```python
from build123d import *

# Parameters (mm, degrees)
CROQUIS4_OUTSIDE_W    = 60.478
CROQUIS4_OUTSIDE_H    = 60.478
CORTAR_EXTRUIR6_DEPTH = 70
CROQUIS5_OUTSIDE_W    = 188.422
CROQUIS5_OUTSIDE_H    = 183.78
CROQUIS5_OUTSIDE_R    = 15
CORTAR_EXTRUIR7_DEPTH = 70
CORTAR_EXTRUIR7_TAPER = 45
CROQUIS6_R            = 9
CORTAR_EXTRUIR8_DEPTH = 15
CHAFL_N1_SIZE         = 2
REDONDEO1_R           = 1
CROQUIS7_OUTSIDE_W    = 83.062
CROQUIS7_OUTSIDE_H    = 78.42
CROQUIS7_OUTSIDE_R    = 15
CORTAR_EXTRUIR9_DEPTH = 10
CORTAR_EXTRUIR9_TAPER = 60


with BuildPart() as part:
    # Croquis1 → Revolución1 (revolve)
    with BuildSketch(Plane.XY):
        Polygon((6.35, 31.379194031), (20, 31.379194031), (22, 31.379194031), (22, 29.379194031), (22, 14.379194031), (22, 12.379194031), (20, 12.379194031), (14, 12.379194031), (11.11, 12.379194031), (11.11, 9.379194031), (9.525, -5.620805969), (1.5875, -5.620805969), (1.5875, 12.379194031), (6.35, 12.379194031), align=None)
    revolve(axis=Axis((0, 51.930492424, 0), (0, -1, 0)))

    # Croquis4 outside → Cortar-Extruir6 (cut)
    with BuildSketch(Plane(origin=(0, 31.379194031, 0), x_dir=(1, 0, 0), z_dir=(0, 1, 0))):
        Rectangle(CROQUIS4_OUTSIDE_W, CROQUIS4_OUTSIDE_H)
        Polygon((17.320508076, 0), (8.660254038, 15), (-8.660254038, 15), (-17.320508076, 0), (-8.660254038, -15), (8.660254038, -15), align=None, mode=Mode.SUBTRACT)
    extrude(amount=-CORTAR_EXTRUIR6_DEPTH, mode=Mode.SUBTRACT)

    # Croquis5 outside → Cortar-Extruir7 (cut)
    with BuildSketch(Plane(origin=(0, 31.379194031, 0), x_dir=(1, 0, 0), z_dir=(0, 1, 0))):
        Rectangle(CROQUIS5_OUTSIDE_W, CROQUIS5_OUTSIDE_H)
        Circle(CROQUIS5_OUTSIDE_R, mode=Mode.SUBTRACT)
    extrude(amount=-CORTAR_EXTRUIR7_DEPTH, taper=CORTAR_EXTRUIR7_TAPER, mode=Mode.SUBTRACT)

    # Croquis6 → Cortar-Extruir8 (cut)
    with BuildSketch(Plane(origin=(0, 31.379194031, 0), x_dir=(1, 0, 0), z_dir=(0, 1, 0))):
        Circle(CROQUIS6_R)
    extrude(amount=-CORTAR_EXTRUIR8_DEPTH, mode=Mode.SUBTRACT)

    # Chaflán1
    chafl_n1_edges = [part.edges().sort_by_distance(p)[0] for p in [
        (-9, 31.379194031, 0),
    ]]
    chamfer(chafl_n1_edges, length=CHAFL_N1_SIZE)

    # Redondeo1
    redondeo1_edges = [part.edges().sort_by_distance(p)[0] for p in [
        (-6.35, 16.379194031, 0),
    ]]
    fillet(redondeo1_edges, radius=REDONDEO1_R)

    # Croquis7 outside → Cortar-Extruir9 (cut)
    with BuildSketch(Plane.XZ.offset(-12.379194031)):
        Rectangle(CROQUIS7_OUTSIDE_W, CROQUIS7_OUTSIDE_H)
        Circle(CROQUIS7_OUTSIDE_R, mode=Mode.SUBTRACT)
    extrude(amount=-CORTAR_EXTRUIR9_DEPTH, taper=CORTAR_EXTRUIR9_TAPER, mode=Mode.SUBTRACT)


solid = part.part
```
Part model, mm, in its own coordinate system. A direction names the side the tool comes from. Round coordinates to 2 decimals unless told otherwise and drop trailing zeros. Loops run counter-clockwise (first coordinate to the right, second up) from the corner with the lowest first, then second, coordinate; pieces in that order, holes last. Notation, with made-up numbers: (42, 65.25) -> (90, 65.25) arc R21 ccw to (90, 89.25) -> close; hole circle Ø6 at (-29, 89). An arc over 180 degrees is marked (long way). Use CSV: the item, a comma, the result in double quotes. Start each with the question number.
1) Cut at C-C, the plane y = -3. Write the cut outline in (x, z) (1 decimal).
2) Wall check: L1, parallel to Z at x = 0, y = 14.4; L2, parallel to X at y = 26, z = 0; L3, parallel to X at y = 14, z = 0. Give the ranges that are in metal, low to high. Write a range as [from, to].
3) Drop flat-ended pins along their axis: P1, Ø2, axis at x = -5.5, y = 6, coming from the -Z side; P2, Ø8, axis at y = 11, z = -9.5, coming from the +X side; P3, Ø3.5, axis at x = 0, z = 0, coming from the +Y side. Give the stop position or say it passes through.
4) Which spindle directions (+Z, -Z, +X, -X, +Y, -Y) get a long thin tool onto all of the face, cutting with end or side? Do faces 1 (the cylindrical face through (-1.38, 13.9, -6.2)), 2 (the cylindrical face through (-8.817, 10.858, -6.76)), 3 (the conical face through (-7.749, 30.815, 13.498)). Say none if no direction does.
5) Cut at B-B, the plane y = 3.5. Write the cut outline in (x, z) (1 decimal).
6) Cut at A-A, the plane y = 21. Write the cut outline in (x, z), plus the area to 3 significant figures.
7) Pull direction X, two halves, no side cores. Call faces 4 (the flat face through (0, 22, 15)), 5 (the conical face through (-2.2, 0.11, -9.89)), 6 (the cylindrical face through (-1.172, 22.97, -8.923)): +X half, -X half, draft (parallel to the pull), parting line (faces both ways), or undercut.
Determined:
1,outline,"circle Ø19.6 at (0, 0); hole circle Ø3.2 at (0, 0)"
2,L1,"z = [-15, -6.35], [6.35, 15]"
2,L2,"x = [-17.32, -9], [9, 17.32]"
2,L3,"x = [-17.32, -6.35], [6.35, 17.32]"
3,P1,"stops at z = -9.78"
3,P2,"stops at x = 13.99"
3,P3,"stops at y = 12.38"
4,face 1,"+Y"
4,face 2,"-Y"
4,face 3,"+Z, -X, +Y"
5,outline,"circle Ø21 at (0, 0); hole circle Ø3.2 at (0, 0)"
6,outline,"(-17.32, 0) -> (-8.66, -15) -> (8.66, -15) -> (17.32, 0) -> (8.66, 15) -> (-8.66, 15) -> close; hole circle Ø18 at (0, 0)"
6,area,"525 mm2"
7,face 4,"draft"
7,face 5,"parting line"
7,face 6,"undercut"
